from build123d import *

# Parameters (mm, degrees)
F1_DEPTH = 1054.1
F3_DEPTH = 152.4
F4_W     = 1178.906798
F4_H     = 114.3
F5_DEPTH = 1270
F7_DEPTH = 25.4


with BuildPart() as f1:
    # F0 (on Top) → F1 (new body)
    with BuildSketch(Plane.XY):
        Polygon((609.6, 57.15), (609.6, 76.2), (-609.6, 76.2), (-609.6, 57.15), (-608.838, 57.15), (-608.838, -57.15), (-609.6, -57.15), (-609.6, -76.2), (609.6, -76.2), (609.6, -57.15), (608.838, -57.15), (608.838, 57.15), align=None)
    extrude(amount=F1_DEPTH)

    # F2 (on face) → F3 (cut)
    with BuildSketch(Plane.XZ.offset(76.2)):
        Polygon((-228.6, 101.6), (0, 101.6), (228.6, 101.6), (228.6, 558.8), (-228.6, 558.8), align=None)
    extrude(amount=-F3_DEPTH, mode=Mode.SUBTRACT)

    # F4 (on face) → F5 (cut)
    with BuildSketch(Plane.XY.offset(1054.1)):
        Rectangle(F4_W, F4_H)
    extrude(amount=-F5_DEPTH, mode=Mode.SUBTRACT)

    # F6 (on face) → F7 (cut)
    with BuildSketch(Plane.XZ.offset(76.2)):
        with BuildLine():
            ThreePointArc((0, 1020.7625), (-21.328108, 969.271892), (30.1625, 990.6))
            ThreePointArc((30.1625, 990.6), (21.328108, 1011.928108), (0, 1020.7625))
        make_face()
    extrude(amount=-F7_DEPTH, mode=Mode.SUBTRACT)


solid = f1.part
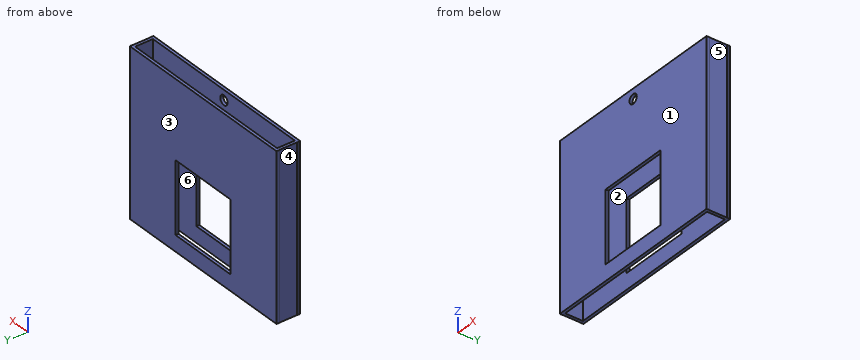
Could you check a few things on this model? Use its own coordinates, in mm. Face numbers are marked on the shaded views. A direction names the side the tool comes from. Give positions to 0.01 mm unless a question says otherwise; leave off trailing zeros. Order: outer loops, then holes, each group sorted by start corner. A loop starts at its lowest first (then second) coordinate and runs counter-clockwise, first axis right, second up. Notation, with made-up numbers: (8, 10.25) - (27, 10.25) arc R14 cw to (27, 14.25) - close; hole circle Ø6 at (75.5, 69). An arc over 180 degrees is marked (long way). Return JSON: item names as keys, results as strings. Group by question number.
Q1. Suppose I cut it at C-C, the plane y = 7. Please give me the cut outline in (x, z).
Q2. Which directions (+Z, -Z, +X, -X, +Y, -Y) give clear straight access to the entire face, cutting with the end or side of a thin tool? Please do the marked faces 1 and 2.
Q3. Will these pins go through, and if not, where does the flat tip stop? pin 1 Ø1 at (y, z) = (0.5, 831) entering from -X; pin 2 Ø4 at (y, z) = (20.5, 846) entering from +X; pin 3 Ø5.5 at (x, y) = (107.5, 68) entering from -Z.
Q4. Thinking about a two-plate mould opening in X: for the marked faces 3, 4, 5 and 6, which applies, pulls with the +X half, pulls with the -X half, needs draft (parallel to the pull), parting line crosses it, or undercut?
Q5. Suppose I cut it at D-D, the plane x = 517. Please give me the cut outline in (y, z), and give its area (3 significant figures).
Q6. Suppose I cut it at A-A, the plane z = 866.5. Please give me the cut outline in (x, y).
Q7. Please list where these lines run through material, in increasing order: line 1 along Y through (x, z) = (60, 787.5); line 2 along X through (y, z) = (-66, 990.6). Write a range as [from, to].
Q8. Suppose I cut it at B-B, the plane x = -110. Please give me the cut outline in (y, z), and give its area (3 significant figures).
Resolved:
{
 "1": {"outline": "(-608.84, 0) - (-589.45, 0) - (-589.45, 1054.1) - (-608.84, 1054.1) - close; (589.45, 0) - (608.84, 0) - (608.84, 1054.1) - (589.45, 1054.1) - close"},
 "2": {"face 1": "+Z, -Z, +X, -X, -Y", "face 2": "+Z, -Z"},
 "3": {"pin 1": "stops at x = -608.84", "pin 2": "stops at x = 608.84", "pin 3": "stops at z = 0"},
 "4": {"face 3": "needs draft", "face 4": "pulls with the -X half", "face 5": "pulls with the +X half", "face 6": "undercut"},
 "5": {"outline": "(-76.2, 0) - (-57.15, 0) - (-57.15, 1054.1) - (-76.2, 1054.1) - close; (57.15, 0) - (76.2, 0) - (76.2, 1054.1) - (57.15, 1054.1) - close", "area": "40,200 mm2"},
 "6": {"outline": "(-609.6, -76.2) - (609.6, -76.2) - (609.6, -57.15) - (608.84, -57.15) - (608.84, 57.15) - (609.6, 57.15) - (609.6, 76.2) - (-609.6, 76.2) - (-609.6, 57.15) - (-608.84, 57.15) - (-608.84, -57.15) - (-609.6, -57.15) - close; hole (-589.45, -57.15) - (589.45, -57.15) - (589.45, 57.15) - (-589.45, 57.15) - close"},
 "7": {"line 1": "y = [-76.2, -57.15], [57.15, 76.2]", "line 2": "x = [-609.6, -30.16], [30.16, 609.6]"},
 "8": {"outline": "(-76.2, 0) - (-57.15, 0) - (-57.15, 101.6) - (-76.2, 101.6) - close; (-76.2, 558.8) - (-57.15, 558.8) - (-57.15, 1054.1) - (-76.2, 1054.1) - close; (57.15, 0) - (76.2, 0) - (76.2, 101.6) - (57.15, 101.6) - close; (57.15, 558.8) - (76.2, 558.8) - (76.2, 1054.1) - (57.15, 1054.1) - close", "area": "22,700 mm2"}
}
